from build123d import *

# Parameters (mm, degrees)
F0_R     = 27.153692
F1_DEPTH = 158.496
F3_DEPTH = 6.35
F4_COUNT = 8


with BuildPart() as f1:
    # F0 (on Top) → F1 (new body)
    with BuildSketch(Plane.XY):
        Circle(F0_R)
    extrude(amount=F1_DEPTH)

    # F2 (on Right) → F3 (join, symmetric)
    with BuildSketch(Plane.YZ):
        Polygon((6.657729, 76.2), (6.657729, 0), (74.554974, 0), align=None)
    extrude(amount=F3_DEPTH, both=True)



with BuildPart() as f4_1:
    # F4: instance of F1
    add(f1.part.rotate(Axis((0, 0, 0), (0, 0, -1)), 1 * 360 / F4_COUNT))


with BuildPart() as f4_2:
    # F4: instance of F1
    add(f1.part.rotate(Axis((0, 0, 0), (0, 0, -1)), 2 * 360 / F4_COUNT))


with BuildPart() as f4_3:
    # F4: instance of F1
    add(f1.part.rotate(Axis((0, 0, 0), (0, 0, -1)), 3 * 360 / F4_COUNT))


with BuildPart() as f4_4:
    # F4: instance of F1
    add(f1.part.rotate(Axis((0, 0, 0), (0, 0, -1)), 4 * 360 / F4_COUNT))


with BuildPart() as f4_5:
    # F4: instance of F1
    add(f1.part.rotate(Axis((0, 0, 0), (0, 0, -1)), 5 * 360 / F4_COUNT))


with BuildPart() as f4_6:
    # F4: instance of F1
    add(f1.part.rotate(Axis((0, 0, 0), (0, 0, -1)), 6 * 360 / F4_COUNT))


with BuildPart() as f4_7:
    # F4: instance of F1
    add(f1.part.rotate(Axis((0, 0, 0), (0, 0, -1)), 7 * 360 / F4_COUNT))


with BuildPart() as f1_1:
    add(f1.part)

    add(f4_1.part)  # F6 merges F4_1

    add(f4_2.part)  # F6 merges F4_2

    add(f4_3.part)  # F6 merges F4_3

    add(f4_4.part)  # F6 merges F4_4

    add(f4_5.part)  # F6 merges F4_5

    add(f4_6.part)  # F6 merges F4_6

    add(f4_7.part)  # F6 merges F4_7
    # F5 (on Right) → F6 (revolve)
    with BuildSketch(Plane.YZ):
        Polygon((-25.58529, 154.478967), (0, 154.478967), (0, 202.92218), align=None)
    revolve(axis=Axis((0, 0, 178.700574), (0, 0, 1)))


solid = f1_1.part
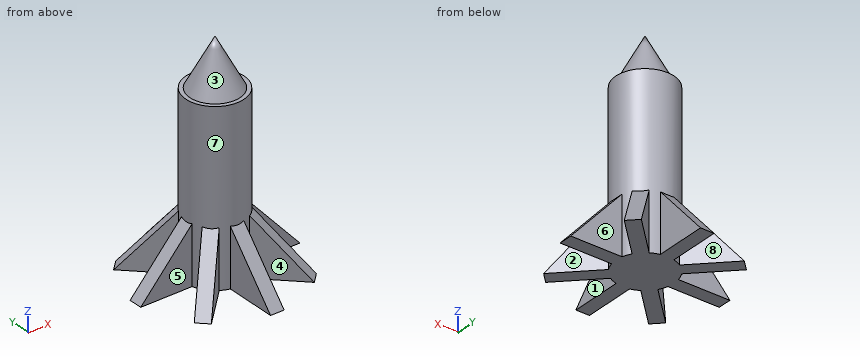
Read the model definition and answer for the solid it produces. Units are mm, in the model's axes. Face numbers are marked on the shaded views. A direction names the side the tool comes from. Round coordinates to 2 decimals unless told otherwise and drop trailing zeros. Loops run counter-clockwise (first coordinate to the right, second up) from the corner with the lowest first, then second, coordinate; pieces in that order, holes last.
Q1. Section A-A on x = -34 is taken. Write down the section's boundary in (y, z).
Q2. Each of these flat-tipped pins is pushed along its axis until it touches: pin 1 (8 mm diameter, centred on y = 28.5, z = 135.5, fed in from -X); pin 2 (4 mm diameter, centred on x = -6, y = -1, fed in from +Z); pin 3 (6 mm diameter, centred on x = 5, y = -4.5, fed in from +Z). Where does it stop, or does it pass through?
Q3. Which of the six approach directions +Z, -Z, +X, -X, +Y, -Y give full straight-line access (tool end or side, diameter ignored) to the marked faces 4, 5, 6, 7 and 8?
Q4. Section C-C on y = 31.5 is taken. Write down the section's boundary in (x, z), and give its area (3 significant figures).
Q5. Determine the mould class of the marked faces 1, 2 and 3 for opening direction X: released by +X, released by -X, zero draft, split by the parting line, or undercut.
Q6. Consider probe 1 along Y at (x, z) = (-36, 8.5); probe 2 along Y at (x, z) = (19, 118.5); probe 3 along X at (y, z) = (-23, 128.5). Determine where each line is inside the solid, lowest interval first.
Output:
1. outline: (-42.98, 0) - (-25.02, 0) - (-25.02, 36.84) - (-42.98, 22.58) - close; (-6.35, 0) - (6.35, 0) - (6.35, 45.51) - (-6.35, 45.51) - close; (25.02, 0) - (42.98, 0) - (42.98, 22.58) - (25.02, 36.84) - close
2. pin 1: stops at x = -11.71
2. pin 2: stops at z = 195.19
2. pin 3: stops at z = 195.87
3. face 4: +Z, -Z, -Y
3. face 5: +Z, -Z, -X
3. face 6: +Z, -Z, +X
3. face 7: +Z
3. face 8: +Z, -Z, +Y
4. outline: (-40.48, 0) - (-22.52, 0) - (-22.52, 40.8) - (-40.48, 26.55) - close; (-6.35, 0) - (6.35, 0) - (6.35, 48.32) - (-6.35, 48.32) - close; (22.52, 0) - (40.48, 0) - (40.48, 26.55) - (22.52, 40.8) - close
4. area: 1,820 mm2
5. face 1: undercut
5. face 2: released by +X
5. face 3: split by the parting line
6. probe 1: y = -44.98 to -27.02, -6.35 to 6.35, 27.02 to 44.98
6. probe 2: y = -19.4 to 19.4
6. probe 3: x = -14.43 to 14.43
